from build123d import *

# Parameters (mm, degrees)
F1_DEPTH = 71
F3_D     = 4


# Not quite as in the source:
# - ends of sketch curves that miss each other by under 0.0002 mm in the source are joined


with BuildPart() as f1:
    # F0 (on Front) → F1 (new body)
    with BuildSketch(Plane.XZ):
        with BuildLine():
            Line((8.1618498422, -10.3647895785), (9.4053820611, -11.6083214649))
            Line((9.4053820611, -11.6083214649), (9.415382064, -11.6183214649))
            Line((9.415382064, -11.6183214649), (20.6153802021, -11.6183214651))
            Line((20.6153802021, -11.6183214651), (22.165411006, -10.0682906612))
            Line((22.165411006, -10.0682906612), (22.1654110059, -7.3944052326))
            Line((22.1654110059, -7.3944052326), (22.1654110059, 3.7817118842))
            Line((22.1654110059, 3.7817118842), (30.0405793841, 3.7817118842))
            Line((30.0405793841, 3.7817118842), (30.515407573, 3.7817104728))
            Line((30.515407573, 3.7817104728), (31.5154075725, 4.7816793802))
            Line((31.5154075725, 4.7816793802), (31.5153703792, 12.7817118841))
            Line((31.5153703792, 12.7817118841), (30.5153417686, 13.7816508489))
            Line((30.5153417686, 13.7816508489), (16.9153093619, 13.7816508489))
            Line((16.9153093619, 13.7816508489), (16.7618646746, 13.6281611659))
            ThreePointArc((16.7618646746, 13.6281611659), (16.5996530095, 13.5197747929), (16.4083113037, 13.4817145544))
            Line((16.4083113037, 13.4817145544), (8.422430452, 13.4817145544))
            ThreePointArc((8.422430452, 13.4817145544), (8.2310887291, 13.5197747818), (8.0688770472, 13.6281611561))
            Line((8.0688770472, 13.6281611561), (7.9153584589, 13.7816508489))
            Line((7.9153584589, 13.7816508489), (-8.0846315282, 13.7816508491))
            Line((-8.0846315282, 13.7816508491), (-8.2381152983, 13.628161166))
            ThreePointArc((-8.2381152983, 13.628161166), (-8.4003269909, 13.5197747816), (-8.5916687288, 13.4817145545))
            Line((-8.5916687288, 13.4817145545), (-16.5775495805, 13.4817145545))
            ThreePointArc((-16.5775495805, 13.4817145545), (-16.7688912713, 13.5197747934), (-16.9311029256, 13.6281611562))
            Line((-16.9311029256, 13.6281611562), (-17.0845685953, 13.7816508491))
            Line((-17.0845685953, 13.7816508491), (-30.4846162694, 13.7816508492))
            Line((-30.4846162694, 13.7816508492), (-31.4846296209, 12.7816374978))
            Line((-31.4846296209, 12.7816374978), (-31.4846296209, 4.7816793804))
            Line((-31.4846296209, 4.7816793804), (-30.4846296214, 3.781710473))
            Line((-30.4846296214, 3.781710473), (-30.0098014316, 3.7817118844))
            Line((-30.0098014316, 3.7817118844), (-22.1346330541, 3.781710473))
            Line((-22.1346330541, 3.781710473), (-22.1346330541, -7.3944052328))
            Line((-22.1346330541, -7.3944052328), (-22.134633054, -10.068299435))
            Line((-22.134633054, -10.068299435), (-20.5846110242, -11.6183214649))
            Line((-20.5846110242, -11.6183214649), (-9.3846416371, -11.618321465))
            Line((-9.3846416371, -11.618321465), (-9.3746416371, -11.6083214649))
            Line((-9.3746416371, -11.6083214649), (-8.1310434239, -10.3647232516))
            ThreePointArc((-8.1310434239, -10.3647232516), (-8.0226570482, -10.2025115772), (-7.9845968145, -10.011169861))
            Line((-7.9845968145, -10.011169861), (-7.9845968145, -5.9254873742))
            ThreePointArc((-7.9845968145, -5.9254873742), (-8.0226567217, -5.7341464462), (-8.1310422173, -5.5719351901))
            Line((-8.1310422173, -5.5719351901), (-8.2697056959, -5.4332707651))
            ThreePointArc((-8.2697056959, -5.4332707651), (-8.3164840652, -5.3595306247), (-8.3273828922, -5.2728874501))
            ThreePointArc((-8.3273828922, -5.2728874501), (-8.6904695936, -4.0063582713), (-9.8182893525, -3.3252190015))
            ThreePointArc((-9.8182893525, -3.3252190015), (-9.9374803464, -3.2570419887), (-9.9846168416, -3.1280739736))
            Line((-9.9846168416, -3.1280739736), (-9.9846168416, -1.6015777605))
            ThreePointArc((-9.9846168416, -1.6015777605), (-9.9374803464, -1.4726097454), (-9.8182893525, -1.4044327326))
            ThreePointArc((-9.8182893525, -1.4044327326), (-8.8323144095, -0.8871586543), (-8.3383526746, 0.1106994843))
            ThreePointArc((-8.3383526746, 0.1106994843), (-8.2712261249, 0.2330065304), (-8.1404708137, 0.2816689983))
            Line((-8.1404708137, 0.2816689983), (8.1712371304, 0.2816689983))
            ThreePointArc((8.1712371304, 0.2816689983), (8.3019924416, 0.2330065304), (8.3691189913, 0.1106994843))
            ThreePointArc((8.3691189913, 0.1106994843), (8.8630871156, -0.8871651956), (9.8490736962, -1.4044358116))
            ThreePointArc((9.8490736962, -1.4044358116), (9.968266036, -1.4726123905), (10.0154031856, -1.6015811811))
            Line((10.0154031856, -1.6015811811), (10.0154031856, -3.1280705531))
            ThreePointArc((10.0154031856, -3.1280705531), (9.968266036, -3.2570393436), (9.8490736962, -3.3252159226))
            ThreePointArc((9.8490736962, -3.3252159226), (8.7212476918, -4.0063428806), (8.3581472677, -5.2728670656))
            ThreePointArc((8.3581472677, -5.2728670656), (8.3472477253, -5.3595093685), (8.3004693733, -5.4332486014))
            Line((8.3004693733, -5.4332486014), (8.161849795, -5.5718681798))
            ThreePointArc((8.161849795, -5.5718681798), (8.0534634193, -5.7340798542), (8.0154031856, -5.9254215704))
            Line((8.0154031856, -5.9254215704), (8.0154031855, -10.0112361406))
            ThreePointArc((8.0154031855, -10.0112361406), (8.0534634321, -10.2025778877), (8.1618498422, -10.3647895785))
        make_face()
    extrude(amount=F1_DEPTH)

    # F3 (through all)
    with Locations(Plane(origin=(0, 0, 0.2816689983), x_dir=(1, 0, 0), z_dir=(0, 0, -1))):
        with Locations((-26.4846296209, 55.5), (26.5153703791, 55.5), (26.5153703791, 15.5), (-26.4846296209, 15.5)):
            Hole(F3_D / 2)


solid = f1.part
Can you work these out from the model? Positions are in its coordinate system, mm. A direction names the side the tool comes from. Round coordinates to 2 decimals unless told otherwise and drop trailing zeros. Order: outer loops, then holes, each group sorted by start corner. A loop starts at its lowest first (then second) coordinate and runs counter-clockwise, first axis right, second up. Notation, with made-up numbers: (-7.5, 58) -> (39.5, 58) arc R20 cw to (39.5, 74) -> close; hole circle Ø4 at (61, 10.5). An arc over 180 degrees is marked (long way). Write each question's results on one line, items separated by ' | '. Start each with the question number.
Item 1: Which directions (+Z, -Z, +X, -X, +Y, -Y) give clear straight access to the entire face, cutting with the end or side of a thin tool? Please do faces 1 (the cylindrical face through (8.852, -35.003, -0.876)), 2 (the flat face through (-21.37, -35.003, -10.832)), 3 (the flat face through (8.015, -35, -8)), 4 (the flat face through (-13, -35, 13.482)).
Item 2: If we section it at A-A, the plane x = 27.5: Write out the boundary of the cut face in (y, z).
Item 3: Please list where these lines run through material, in increasing order: L1, parallel to X at y = -15.5, z = 6; L2, parallel to X at y = -27, z = -9.5; L3, parallel to Y at x = 27, z = 11.
Item 4: Will these pins go through, and if not, where does the flat tip stop? pin 1 (6.5 mm diameter, centred on x = 27.5, y = -41.5, fed in from -Z); pin 2 (1.2 mm diameter, centred on y = -38.5, z = -2, fed in from +X); pin 3 (10 mm diameter, centred on y = -35, z = -3.5, fed in from -X); pin 4 (6.5 mm diameter, centred on x = -26.48, y = -55.5, fed in from +Z).
Item 5: If we section it at B-B, the plane x = 2.5: Write out the boundary of the cut face in (y, z), then the cut area to 4 significant figures.
Item 6: Thinking about a two-plate mould opening in Z: for faces 5 (the flat face through (-7.985, -35, -8)), 6 (the flat face through (-15, -35, -11.618)), 7 (the cylindrical face through (-8.68, -35, -4.02)), which applies, +Z half, -Z half, draft (parallel to the pull), parting line (faces both ways), or undercut?
Item 7: If we section it at C-C, the plane y = -55.5: State how many separate pieces and enclosed holes the cut face has, then the cut area to 3 significant figures.
Results:
1) face 1: +Y, -Y | face 2: -Z, -X, +Y, -Y | face 3: -Z, +Y, -Y | face 4: +Z, +Y, -Y
2) outline: (-71, 3.78) -> (-57.24, 3.78) -> (-57.24, 13.78) -> (-71, 13.78) -> close; (-53.76, 3.78) -> (-17.24, 3.78) -> (-17.24, 13.78) -> (-53.76, 13.78) -> close; (-13.76, 3.78) -> (0, 3.78) -> (0, 13.78) -> (-13.76, 13.78) -> close
3) L1: x = -31.48 to -28.48, -24.48 to 24.52, 28.52 to 31.52 | L2: x = -22.13 to -7.98, 8.02 to 22.17 | L3: y = -71 to -57.44, -53.56 to -17.44, -13.56 to 0
4) pin 1: stops at z = 3.78 | pin 2: stops at x = 22.17 | pin 3: stops at x = -22.13 | pin 4: stops at z = 13.78
5) outline: (-71, 0.28) -> (0, 0.28) -> (0, 13.78) -> (-71, 13.78) -> close | area: 958.5 mm2
6) face 5: draft | face 6: -Z half | face 7: undercut
7) separate pieces: 3 | enclosed holes: 0 | area: 1,020 mm2
